Could you check a few things on this model? Use its own coordinates, in mm. Coordinates: 2 decimals unless noted, no trailing zeros. Write each loop counter-clockwise with the first axis right and the second up, starting at its lowest first coordinate (ties: lowest second). Pieces come first, ordered by that corner, then holes. Notation, with made-up numbers: M 27,9 L 41,9 A27 cw 41,47 Z; hole C 0,-33.75 d2. An arc over 180 degrees is marked long. Answer as CSV lines item,"result". Start each with the question number.
Item 1: Suppose I cut it at C-C, the plane x = 2.75. Write out the boundary of the cut face in (y, z), and give its area (3 significant figures).
Item 2: Suppose I cut it at D-D, the plane y = -1.3. Write out the boundary of the cut face in (x, z), and give its area (3 significant figures).
Item 3: Suppose I cut it at B-B, the plane y = 0. Write out the boundary of the cut face in (x, z).
Item 4: I'm going to push flat-ended pins straight in: P1, Ø2, axis at x = -0.5, z = -3.5, coming from the -Y side; P2, Ø4, axis at x = 3, z = 0.5, coming from the -Y side. Where does each tip first touch, or does it pass through?
Item 5: Suppose I cut it at A-A, the plane z = 1. Write out the boundary of the cut face in (x, y), and give its area (3 significant figures).
Item 6: If I drill on line 1 along Z through (x, y) = (-0.25, 0.9); line 2 along X through (y, z) = (-0.2, 7); line 3 along X through (y, z) = (0.35, 3.5), over which ranges is the centre line in solid material (lowest first)? Write a range as [from, to].
```python
from build123d import *

# Parameters (mm, degrees)
SKETCH2_R           = 2.1
RESISTOR_BODY_DEPTH = 12.1
LEAD1_PROFILE_R     = 0.4
SKETCH6_R           = 0.4
LEAD2_DEPTH         = 7.9


with BuildPart() as part:
    # Sketch2 → Resistor Body (new body)
    with BuildSketch(Plane.XY):
        Circle(SKETCH2_R)
    extrude(amount=RESISTOR_BODY_DEPTH)

    # Lead1: sweep along a path in Lead1 Path
    with BuildLine(Plane(origin=(0, 0, 0), x_dir=(1, 0, 0), z_dir=(0, 1, 0))) as lead1_path:
        Line((0, -12.1), (0, -15.1))
        ThreePointArc((0, -15.1), (0.585786438, -16.514213562), (2, -17.1))
        Line((2, -17.1), (3, -17.1))
        ThreePointArc((3, -17.1), (4.414213562, -16.514213562), (5, -15.1))
        Line((5, -15.1), (5, 7.9))
    # Lead1 Profile → Lead1 (sweep)
    with BuildSketch(Plane(origin=(0, 0, 12.1), x_dir=(-1, 0, 0), z_dir=(0, 0, 1))):
        Circle(LEAD1_PROFILE_R)
    sweep(path=lead1_path.line)

    # Sketch6 → Lead2 (add)
    with BuildSketch(Plane(origin=(0, 0, 0), x_dir=(1, 0, 0), z_dir=(0, 0, -1))):
        Circle(SKETCH6_R)
    extrude(amount=LEAD2_DEPTH)


solid = part.part
```
Ans:
1,outline,"C 0,17.1 d0.8"
1,area,"0.503 mm^2"
2,outline,"M -1.65,0 L 1.65,0 L 1.65,12.1 L -1.65,12.1 Z"
2,area,"39.9 mm^2"
3,outline,"M -2.1,0 L -0.4,0 L -0.4,-7.9 L 0.4,-7.9 L 0.4,0 L 2.1,0 L 2.1,12.1 L 0.4,12.1 L 0.4,15.1 A1.6 cw 2,16.7 L 3,16.7 A1.6 cw 4.6,15.1 L 4.6,-7.9 L 5.4,-7.9 L 5.4,15.1 A2.4 ccw 3,17.5 L 2,17.5 A2.4 ccw -0.4,15.1 L -0.4,12.1 L -2.1,12.1 Z"
4,P1,"stops at y = -0.4"
4,P2,"stops at y = -1.85"
5,outline,"C 0,0 d4.2; C 5,0 d0.8"
5,area,"14.4 mm^2"
6,line 1,"z = [0, 12.1]"
6,line 2,"x = [-2.09, 2.09], [4.65, 5.35]"
6,line 3,"x = [-2.07, 2.07], [4.81, 5.19]"
